from build123d import *

# Parameters (mm, degrees)
SKETCH1_R           = 2.0193
BOSS_EXTRUDE1_DEPTH = 26.9875
SKETCH2_R           = 6.35
SKETCH2_R_2         = 2.0193
BOSS_EXTRUDE2_DEPTH = 7.9375


with BuildPart() as part:
    # Sketch1 → Boss-Extrude1 (new, symmetric)
    with BuildSketch(Plane.XY):
        with BuildLine():
            ThreePointArc((0.93173274, 6.79441227), (0, 6.858), (-0.93173274, 6.79441227))
            Line((-0.93173274, 6.79441227), (-5.41826726, 4.204110358))
            ThreePointArc((-5.41826726, 4.204110358), (-5.939202219, 3.429), (-6.35, 2.590301913))
            Line((-6.35, 2.590301913), (-6.35, -2.590301913))
            ThreePointArc((-6.35, -2.590301913), (-5.939202219, -3.429), (-5.41826726, -4.204110358))
            Line((-5.41826726, -4.204110358), (-0.93173274, -6.79441227))
            ThreePointArc((-0.93173274, -6.79441227), (0, -6.858), (0.93173274, -6.79441227))
            Line((0.93173274, -6.79441227), (5.41826726, -4.204110358))
            ThreePointArc((5.41826726, -4.204110358), (5.939202219, -3.429), (6.35, -2.590301913))
            Line((6.35, -2.590301913), (6.35, 2.590301913))
            ThreePointArc((6.35, 2.590301913), (5.939202219, 3.429), (5.41826726, 4.204110358))
            Line((5.41826726, 4.204110358), (0.93173274, 6.79441227))
        make_face()
        Circle(SKETCH1_R, mode=Mode.SUBTRACT)
    extrude(amount=BOSS_EXTRUDE1_DEPTH, both=True)

    # Sketch2 → Boss-Extrude2 (add)
    with BuildSketch(Plane.XY.offset(26.9875)):
        Circle(SKETCH2_R)
        Circle(SKETCH2_R_2, mode=Mode.SUBTRACT)
    boss_extrude2 = extrude(amount=BOSS_EXTRUDE2_DEPTH)

    # Mirror1: Boss-Extrude2 across plane
    add(boss_extrude2.mirror(Plane.XY))


solid = part.part
Work out the finished part from the listing and answer in its coordinate system (mm). A direction names the side the tool comes from. Round coordinates to 2 decimals unless told otherwise and drop trailing zeros. Write each loop counter-clockwise with the first axis right and the second up, starting at its lowest first coordinate (ties: lowest second). Pieces come first, ordered by that corner, then holes. Notation, with made-up numbers: (12, 68) - (49, 68) arc R18 cw to (49, 89) - close; hole circle Ø11 at (47.25, -37.75). An arc over 180 degrees is marked (long way). Answer in a Markdown table with one row per item. Add a question column.
1. For faces 4 (the flat face through (5.6, -3.3, 26.988)), 5 (the cylindrical face through (-1.38, -6.2, 30.9)), 6 (the flat face through (5.7, 3.2, 26.988)), 7 (the flat face through (-5.7, 3.2, -26.988)), determine the directions among +Z, -Z, +X, -X, +Y, -Y from which every point of the face is accessible in a straight line to the end or side of a thin tool.
2. Given pin 1 (1.5 mm diameter, centred on x = -2, z = -23.5, fed in from +Y); pin 2 (3 mm diameter, centred on x = 0, y = 0, fed in from -Z); pin 3 (2 mm diameter, centred on x = 2, z = -10, fed in from +Y) (3 decimals); pin 4 (1 mm diameter, centred on y = 5.5, z = 2, fed in from +X), each flat-ended and moving along its own axis, determine where each tip first touches the part or whether it passes through.
3. Find the intervals of material crossed by line 1 along Y through (x, z) = (0, -17); line 2 along Y through (x, z) = (0.5, 22.5); line 3 along X through (y, z) = (-1, -13), in increasing order. Write a range as from..to.
4. A cutting plane is placed at B-B, the plane z = -10.5. Determine the outline of the cut face in (x, y), and give its area (3 significant figures).
5. The mould has two halves that part along X. Classify faces 1 (the flat face through (-3.14, 5.52, 0.38)), 2 (the flat face through (0, -6.5, -26.988)), 3 (the cylindrical face through (1.926, 0.607, 0.489)): +X half, -X half, draft (parallel to the pull), parting line (faces both ways), or undercut.
Worked out:
| question | item | result |
|---|---|---|
| 1 | face 4 | +Z, +X, -Y |
| 1 | face 5 | +Z |
| 1 | face 6 | +Z, +X, +Y |
| 1 | face 7 | -Z, -X, +Y |
| 2 | pin 1 | y = 6.61 |
| 2 | pin 2 | through |
| 2 | pin 3 | y = 6.755 |
| 2 | pin 4 | x = 4.04 |
| 3 | line 1 | -6.86..-2.02, 2.02..6.86 |
| 3 | line 2 | -6.84..-1.96, 1.96..6.84 |
| 3 | line 3 | -6.35..-1.75, 1.75..6.35 |
| 4 | outline | (-6.35, -2.59) arc R6.86 ccw to (-5.42, -4.2) - (-0.93, -6.79) arc R6.86 ccw to (0.93, -6.79) - (5.42, -4.2) arc R6.86 ccw to (6.35, -2.59) - (6.35, 2.59) arc R6.86 ccw to (5.42, 4.2) - (0.93, 6.79) arc R6.86 ccw to (-0.93, 6.79) - (-5.42, 4.2) arc R6.86 ccw to (-6.35, 2.59) - close; hole circle Ø4.04 at (0, 0) |
| 4 | area | 124 mm^2 |
| 5 | face 1 | -X half |
| 5 | face 2 | draft |
| 5 | face 3 | undercut |
